```python
from build123d import *

# Parameters (mm, degrees)
F0_W     = 70
F0_H     = 15
F0_R     = 1
F1_DEPTH = 8
F2_SIZE  = 2
F4_DEPTH = 70
F5_R     = 1
F6_R     = 0.5


with BuildPart() as f1:
    # F0 (on Top) → F1 (new body)
    with BuildSketch(Plane.XY):
        with Locations((35, 7.5)):
            Rectangle(F0_W, F0_H)
        with Locations((11, 7.5)):
            Circle(F0_R, mode=Mode.SUBTRACT)
        with Locations((59, 7.5)):
            Circle(F0_R, mode=Mode.SUBTRACT)
    extrude(amount=F1_DEPTH)

    # F2
    f2_edges = [f1.edges().sort_by_distance(p)[0] for p in [
        (10, 7.5, 8),
        (58, 7.5, 8),
    ]]
    chamfer(f2_edges, length=F2_SIZE)

    # F3 (on face) → F4 (join)
    with BuildSketch(Plane.YZ.offset(70)):
        Polygon((50, 8), (15, 8), (15, 0), align=None)
    extrude(amount=-F4_DEPTH)

    # F5
    f5_edges = [f1.edges().sort_by_distance(p)[0] for p in [
        (35, 50, 8),
    ]]
    fillet(f5_edges, radius=F5_R)

    # F6
    f6_edges = [f1.edges().sort_by_distance(p)[0] for p in [
        (35, 0, 8),
    ]]
    fillet(f6_edges, radius=F6_R)


solid = f1.part
```
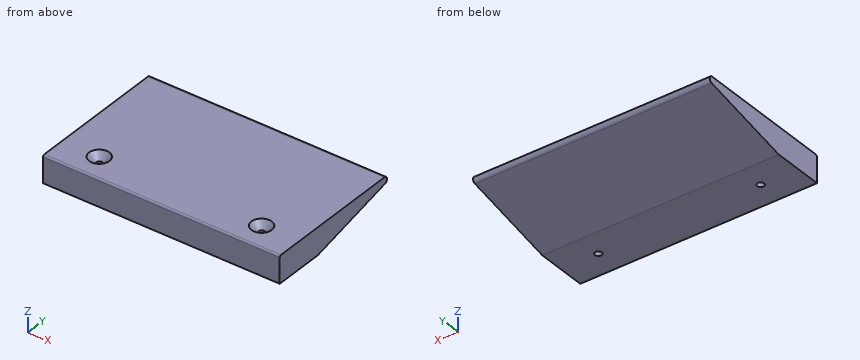
CAD build for the part. Positions are in the model's coordinates, mm. Coordinates: 2 decimals unless noted, no trailing zeros. Order: outer loops, then holes, each group sorted by start corner. A loop starts at its lowest first (then second) coordinate and runs counter-clockwise, first axis right, second up. Notation, with made-up numbers: M -16,59 L 16,59 A27 ccw 16,82 Z; hole C 14,10 d2. An arc over 180 degrees is marked long. Answer as CSV lines item,"result".
1) Flat gauge pins, fed straight in: P1, Ø5, axis at x = 9.5, y = 29, coming from the -Z side; P2, Ø1.8, axis at x = 59, y = 7.5, coming from the -Z side; P3, Ø3, axis at x = 11, y = 7.5, coming from the +Z side. Where does each tip first touch, or does it go through?
Verdict:
P1,"z = 2.63"
P2,"through"
P3,"z = 6.5"
2) Cut at B-B (x = 11). List the corners of the cut face in (y, z), then the cut area to 3 significant figures.
Verdict:
outline,"M 0,0 L 6.5,0 L 6.5,6 L 4.5,8 L 0.5,8 A0.5 ccw 0,7.5 Z; M 8.5,0 L 15,0 L 41.36,6.03 A1 ccw 41.14,8 L 10.5,8 L 8.5,6 Z"
area,"233 mm2"
3) Cut at D-D (x = 42.5). List the corners of the cut face in (y, z).
Verdict:
outline,"M 0,0 L 15,0 L 41.36,6.03 A1 ccw 41.14,8 L 0.5,8 A0.5 ccw 0,7.5 Z"
4) Drill centre lines: L1, parallel to Y at x = 60, z = 7.5; L2, parallel to Z at x = 66, y = 37; L3, parallel to Z at x = 3, y = 16. Where is each one in solid material? Low to high. Write a range as from..to.
Verdict:
L1,"0..5.21, 9.79..42"
L2,"5.03..8"
L3,"0.23..8"
5) Cut at A-A (y = 7.5). List the corners of the cut face in (x, z), then the cut area to 3 significant figures.
Verdict:
outline,"M 0,0 L 10,0 L 10,6 L 8,8 L 0,8 Z; M 12,0 L 58,0 L 58,6 L 56,8 L 14,8 L 12,6 Z; M 60,0 L 70,0 L 70,8 L 62,8 L 60,6 Z"
area,"520 mm2"
6) Cut at C-C (z = 4). List the corners of the cut face in (x, y), then the cut area to 3 significant figures.
Verdict:
outline,"M 0,0 L 70,0 L 70,32.5 L 0,32.5 Z; hole C 11,7.5 d2; hole C 59,7.5 d2"
area,"2,270 mm2"
